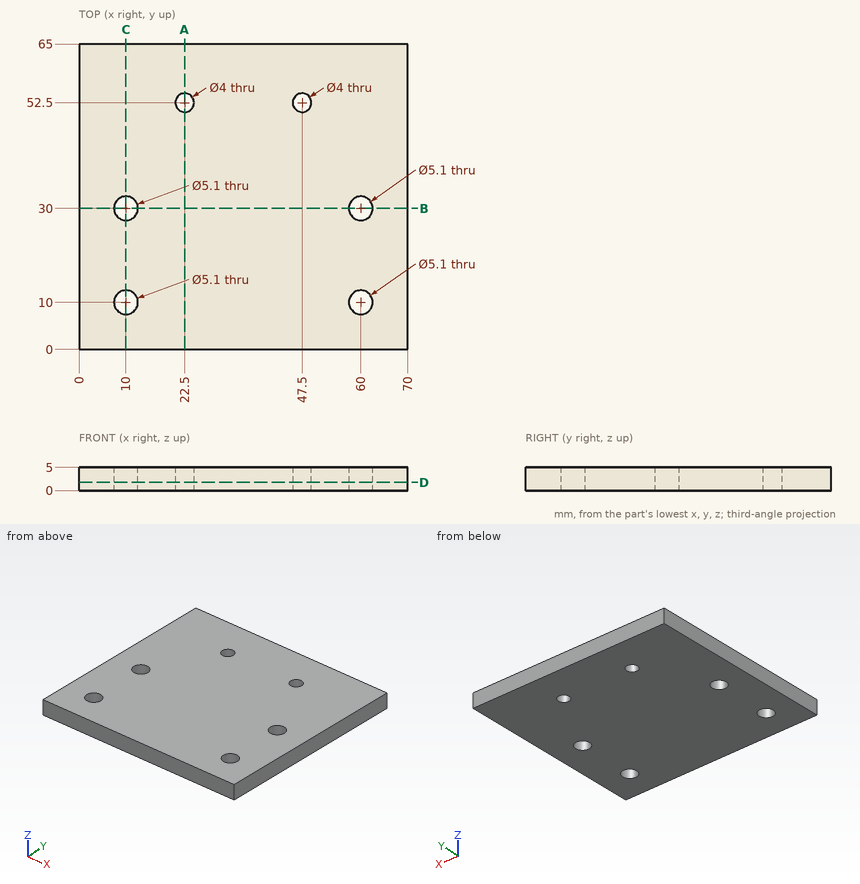
Geometry check sheet. Reference: drawing and pictorial views, mm from the part's lowest x, y, z. Round coordinates to 2 decimals unless told otherwise and drop trailing zeros. Write each loop counter-clockwise with the first axis right and the second up, starting at its lowest first coordinate (ties: lowest second). Pieces come first, ordered by that corner, then holes. Notation, with made-up numbers: (70, -11.5) -> (110, -11.5) arc R8 ccw to (110, 3.5) -> close; hole circle Ø10 at (-2.75, 5). An arc over 180 degrees is marked (long way). Answer as CSV lines item,"result". Start each with the question number.
1) Section check C-C on x = 10. Enter the section's corners in (y, z), and give its area (3 significant figures).
2) Section check B-B on y = 30. Enter the section's corners in (x, z), and give its area (3 significant figures).
3) Material ranges on line 1 (Y direction, x = 60, z = 1.1); line 2 (Y direction, x = 61, z = 0.35); line 3 (Y direction, x = 47.5, z = 3.15), recorded low to high. Write a range as from..to.
4) Section check A-A on x = 22.5. Enter the section's corners in (y, z).
5) Go/stop test with flat-tipped pins: P1, Ø8, axis at x = 10, y = 30, coming from the +Z side; P2, Ø3, axis at x = 22.5, y = 52.5, coming from the +Z side. Record where each tip stops, or that it passes through.
6) Section check D-D on z = 1.8. Enter the section's corners in (x, y), and give its area (3 significant figures).
Found:
1,outline,"(0, 0) -> (7.45, 0) -> (7.45, 5) -> (0, 5) -> close; (12.55, 0) -> (27.45, 0) -> (27.45, 5) -> (12.55, 5) -> close; (32.55, 0) -> (65, 0) -> (65, 5) -> (32.55, 5) -> close"
1,area,"274 mm^2"
2,outline,"(0, 0) -> (7.45, 0) -> (7.45, 5) -> (0, 5) -> close; (12.55, 0) -> (57.45, 0) -> (57.45, 5) -> (12.55, 5) -> close; (62.55, 0) -> (70, 0) -> (70, 5) -> (62.55, 5) -> close"
2,area,"299 mm^2"
3,line 1,"y = 0..7.45, 12.55..27.45, 32.55..65"
3,line 2,"y = 0..7.65, 12.35..27.65, 32.35..65"
3,line 3,"y = 0..50.5, 54.5..65"
4,outline,"(0, 0) -> (50.5, 0) -> (50.5, 5) -> (0, 5) -> close; (54.5, 0) -> (65, 0) -> (65, 5) -> (54.5, 5) -> close"
5,P1,"stops at z = 5"
5,P2,"passes through"
6,outline,"(0, 0) -> (70, 0) -> (70, 65) -> (0, 65) -> close; hole circle Ø5.1 at (10, 10); hole circle Ø5.1 at (10, 30); hole circle Ø4 at (22.5, 52.5); hole circle Ø4 at (47.5, 52.5); hole circle Ø5.1 at (60, 10); hole circle Ø5.1 at (60, 30)"
6,area,"4,440 mm^2"
